CAD build for the part. Positions are in the model's coordinates, mm. A direction names the side the tool comes from. Coordinates: 2 decimals unless noted, no trailing zeros. Order: outer loops, then holes, each group sorted by start corner. A loop starts at its lowest first (then second) coordinate and runs counter-clockwise, first axis right, second up. Notation, with made-up numbers: (-21, 53) - (38, 53) arc R8 cw to (38, 66) - close; hole circle Ø4 at (-7, 68.25). An arc over 180 degrees is marked (long way). Use one line per item in the form item = value.
```python
from build123d import *

# Parameters (mm, degrees)
F0_W     = 82
F0_H     = 48
F0_W_2   = 79
F0_H_2   = 45
F1_DEPTH = 1.5
F2_DEPTH = 11.5


with BuildPart() as f1:
    # F0 (on Front) → F1 (new body)
    with BuildSketch(Plane.XZ):
        Rectangle(F0_W, F0_H)
        Rectangle(F0_W_2, F0_H_2, mode=Mode.SUBTRACT)
        Rectangle(F0_W_2, F0_H_2)
    extrude(amount=F1_DEPTH)

    # F0 (on Front) → F2 (join)
    with BuildSketch(Plane.XZ):
        Rectangle(F0_W, F0_H)
        Rectangle(F0_W_2, F0_H_2, mode=Mode.SUBTRACT)
    extrude(amount=F2_DEPTH)


solid = f1.part
```
Item 1: Cut at A-A, the plane y = -9. Write the cut outline in (x, z), plus the area to 3 significant figures.
Derived:
outline = (-41, -24) - (41, -24) - (41, 24) - (-41, 24) - close; hole (-39.5, -22.5) - (39.5, -22.5) - (39.5, 22.5) - (-39.5, 22.5) - close
area = 381 mm²
Item 2: Cut at B-B, the plane x = 15.5. Write the cut outline in (y, z).
Derived:
outline = (-11.5, -24) - (0, -24) - (0, 24) - (-11.5, 24) - (-11.5, 22.5) - (-1.5, 22.5) - (-1.5, -22.5) - (-11.5, -22.5) - close
Item 3: Cut at C-C, the plane z = -6.5. Write the cut outline in (x, y).
Derived:
outline = (-41, -11.5) - (-39.5, -11.5) - (-39.5, -1.5) - (39.5, -1.5) - (39.5, -11.5) - (41, -11.5) - (41, 0) - (-41, 0) - close
Item 4: Two-plate mould, pull along Z, no slides. Class faces 1 (the face through (39.5, -6, 0)), 2 (the face through (-12, -11.5, -23)), 3 (the face through (-1, -6, 24)): +Z half, -Z half, draft (parallel to the pull), parting line (faces both ways), or undercut.
Derived:
face_1 = undercut
face_2 = draft
face_3 = +Z half
Item 5: Drop a flat-ended pin along its axis: pin 1 (5 mm diameter, centred on x = -28.5, z = 9, fed in from -Y). Give the stop position or say it passes through.
Derived:
pin_1 = -1.5
Item 6: Drill centre lines: line 1 (X direction, y = -1.75, z = 12.5); line 2 (Z direction, x = -11, y = -5.75); line 3 (Y direction, x = 32.5, z = -6). Where is each one in solid material? Low to high. Write a range as [from, to].
Derived:
line_1 = [-41, -39.5], [39.5, 41]
line_2 = [-24, -22.5], [22.5, 24]
line_3 = [-1.5, 0]
Item 7: 3-axis set-ups, long thin cutter, end or side, ignore diameter. For faces 4 (the face through (-1, -6, 22.5)), 5 (the face through (-1, -6, -24)): which of +Z, -Z, +X, -X, +Y, -Y reach the whole face in a straight line?
Derived:
face_4 = -Y
face_5 = -Z, +X, -X, +Y, -Y
